from build123d import *

# Parameters (mm, degrees)
SKETCH1_R            = 10.5
BOSS_EXTRUDE1_DEPTH  = 20
SKETCH2_R            = 12
CUT_EXTRUDE1_DEPTH   = 3
SKETCH3_OUTSIDE_W    = 47.968
SKETCH3_OUTSIDE_H    = 58.968
SKETCH3_OUTSIDE_R    = 19
CUT_EXTRUDE2_DEPTH   = 0.25
SKETCH4_OUTSIDE_W    = 47.968
SKETCH4_OUTSIDE_H    = 58.968
SKETCH4_OUTSIDE_R    = 19
CUT_EXTRUDE3_DEPTH   = 0.25
CUT_EXTRUDE4_DEPTH   = 1.5
LPATTERN1_COUNT      = 6
LPATTERN1_PITCH      = 3
MIRROR1_COPY_1_DEPTH = 1.5
MIRROR1_COPY_2_DEPTH = 1.5
MIRROR1_COPY_3_DEPTH = 1.5
MIRROR1_COPY_4_DEPTH = 1.5
MIRROR1_COPY_5_DEPTH = 1.5
CUT_EXTRUDE5_REACH   = 36
SKETCH6_R            = 4
SKETCH7_R            = 1.5
CUT_EXTRUDE6_DEPTH   = 4
SKETCH9_R            = 1.5
CUT_EXTRUDE7_DEPTH   = 6


with BuildPart() as part:
    # Sketch1 → Boss-Extrude1 (new body)
    with BuildSketch(Plane.XY):
        with BuildLine():
            Line((-17, 14.739402973), (-17, -14.739402973))
            ThreePointArc((-17, -14.739402973), (0, -22.5), (17, -14.739402973))
            Line((17, -14.739402973), (17, 14.739402973))
            ThreePointArc((17, 14.739402973), (0, 22.5), (-17, 14.739402973))
        make_face()
        Circle(SKETCH1_R, mode=Mode.SUBTRACT)
    extrude(amount=BOSS_EXTRUDE1_DEPTH)

    # Sketch2 → Cut-Extrude1 (cut)
    with BuildSketch(Plane.XY.offset(20)):
        Circle(SKETCH2_R)
    extrude(amount=-CUT_EXTRUDE1_DEPTH, mode=Mode.SUBTRACT)

    # Sketch3 outside → Cut-Extrude2 (cut)
    with BuildSketch(Plane(origin=(0, 0, 0), x_dir=(-1, 0, 0), z_dir=(0, 0, -1))):
        Rectangle(SKETCH3_OUTSIDE_W, SKETCH3_OUTSIDE_H)
        Circle(SKETCH3_OUTSIDE_R, mode=Mode.SUBTRACT)
    extrude(amount=-CUT_EXTRUDE2_DEPTH, mode=Mode.SUBTRACT)

    # Sketch4 outside → Cut-Extrude3 (cut)
    with BuildSketch(Plane.XY.offset(20)):
        Rectangle(SKETCH4_OUTSIDE_W, SKETCH4_OUTSIDE_H)
        Circle(SKETCH4_OUTSIDE_R, mode=Mode.SUBTRACT)
    extrude(amount=-CUT_EXTRUDE3_DEPTH, mode=Mode.SUBTRACT)

    # Sketch5 → Cut-Extrude4 (cut)
    with BuildSketch(Plane(origin=(0, 0, 1.75), x_dir=(-1, 0, 0), z_dir=(0, 0, -1))):
        with BuildLine():
            Line((17, 8.485281374), (17, 14.739402973))
            ThreePointArc((17, 14.739402973), (0, 22.5), (-17, 14.739402973))
            Line((-17, 14.739402973), (-17, 8.485281374))
            ThreePointArc((-17, 8.485281374), (0, 19), (17, 8.485281374))
        make_face()
    cut_extrude4 = extrude(amount=-CUT_EXTRUDE4_DEPTH, mode=Mode.SUBTRACT)

    # LPattern1: Cut-Extrude4 ×6
    with Locations(*[(0, 0, i * LPATTERN1_PITCH) for i in range(1, LPATTERN1_COUNT)]):
        add(cut_extrude4, mode=Mode.SUBTRACT)

    # Mirror1: Cut-Extrude4 across plane
    add(cut_extrude4.mirror(Plane.ZX), mode=Mode.SUBTRACT)

    # Mirror1 copy 1 sketch → Mirror1 copy 1 (cut)
    with BuildSketch(Plane(origin=(0, 0, 4.75), x_dir=(-1, 0, 0), z_dir=(0, 0, -1))):
        with BuildLine():
            Line((17, -8.485281374), (17, -14.739402973))
            ThreePointArc((17, -14.739402973), (0, -22.5), (-17, -14.739402973))
            Line((-17, -14.739402973), (-17, -8.485281374))
            ThreePointArc((-17, -8.485281374), (0, -19), (17, -8.485281374))
        make_face()
    extrude(amount=-MIRROR1_COPY_1_DEPTH, mode=Mode.SUBTRACT)

    # Mirror1 copy 2 sketch → Mirror1 copy 2 (cut)
    with BuildSketch(Plane(origin=(0, 0, 7.75), x_dir=(-1, 0, 0), z_dir=(0, 0, -1))):
        with BuildLine():
            Line((17, -8.485281374), (17, -14.739402973))
            ThreePointArc((17, -14.739402973), (0, -22.5), (-17, -14.739402973))
            Line((-17, -14.739402973), (-17, -8.485281374))
            ThreePointArc((-17, -8.485281374), (0, -19), (17, -8.485281374))
        make_face()
    extrude(amount=-MIRROR1_COPY_2_DEPTH, mode=Mode.SUBTRACT)

    # Mirror1 copy 3 sketch → Mirror1 copy 3 (cut)
    with BuildSketch(Plane(origin=(0, 0, 10.75), x_dir=(-1, 0, 0), z_dir=(0, 0, -1))):
        with BuildLine():
            Line((17, -8.485281374), (17, -14.739402973))
            ThreePointArc((17, -14.739402973), (0, -22.5), (-17, -14.739402973))
            Line((-17, -14.739402973), (-17, -8.485281374))
            ThreePointArc((-17, -8.485281374), (0, -19), (17, -8.485281374))
        make_face()
    extrude(amount=-MIRROR1_COPY_3_DEPTH, mode=Mode.SUBTRACT)

    # Mirror1 copy 4 sketch → Mirror1 copy 4 (cut)
    with BuildSketch(Plane(origin=(0, 0, 13.75), x_dir=(-1, 0, 0), z_dir=(0, 0, -1))):
        with BuildLine():
            Line((17, -8.485281374), (17, -14.739402973))
            ThreePointArc((17, -14.739402973), (0, -22.5), (-17, -14.739402973))
            Line((-17, -14.739402973), (-17, -8.485281374))
            ThreePointArc((-17, -8.485281374), (0, -19), (17, -8.485281374))
        make_face()
    extrude(amount=-MIRROR1_COPY_4_DEPTH, mode=Mode.SUBTRACT)

    # Mirror1 copy 5 sketch → Mirror1 copy 5 (cut)
    with BuildSketch(Plane(origin=(0, 0, 16.75), x_dir=(-1, 0, 0), z_dir=(0, 0, -1))):
        with BuildLine():
            Line((17, -8.485281374), (17, -14.739402973))
            ThreePointArc((17, -14.739402973), (0, -22.5), (-17, -14.739402973))
            Line((-17, -14.739402973), (-17, -8.485281374))
            ThreePointArc((-17, -8.485281374), (0, -19), (17, -8.485281374))
        make_face()
    extrude(amount=-MIRROR1_COPY_5_DEPTH, mode=Mode.SUBTRACT)

    # Sketch6 → Cut-Extrude5 (cut, up to next)
    with BuildSketch(Plane.ZY.offset(17), mode=Mode.PRIVATE) as cut_extrude5_sk1:
        with Locations((10, 0)):
            Circle(SKETCH6_R)
    cut_extrude5_tool1 = extrude(cut_extrude5_sk1.sketch, amount=-CUT_EXTRUDE5_REACH, mode=Mode.PRIVATE) & part.part
    add(cut_extrude5_tool1.solids().sort_by_distance((-17, 0, 10))[0], mode=Mode.SUBTRACT)

    # Sketch7 → Cut-Extrude6 (cut)
    with BuildSketch(Plane.ZY.offset(17)):
        with Locations((5.050252532, 4.949747468)):
            Circle(SKETCH7_R)
        with Locations((14.949747468, 4.949747468)):
            Circle(SKETCH7_R)
        with Locations((14.949747468, -4.949747468)):
            Circle(SKETCH7_R)
        with Locations((5.050252532, -4.949747468)):
            Circle(SKETCH7_R)
    cut_extrude6 = extrude(amount=-CUT_EXTRUDE6_DEPTH, mode=Mode.SUBTRACT)

    # Sketch8 → Cut-Revolve1 (revolve, cut)
    with BuildSketch(Plane(origin=(0, 0, 10), x_dir=(-1, 0, 0), z_dir=(0, 0, -1))):
        Polygon((-17, 0), (-17, -3), (-14.5, -3), (-11.5, 0), align=None)
    revolve(axis=Axis((11.5, 0, 10), (1, 0, 0)), mode=Mode.SUBTRACT)

    # Mirror2: Cut-Extrude6 across plane
    add(cut_extrude6.mirror(Plane(origin=(0, 0, 0), x_dir=(0, 0, 1), z_dir=(1, 0, 0))), mode=Mode.SUBTRACT)

    # Sketch9 → Cut-Extrude7 (cut)
    with BuildSketch(Plane(origin=(0, 0, 0), x_dir=(-1, 0, 0), z_dir=(0, 0, -1))):
        with Locations((0, 16)):
            Circle(SKETCH9_R)
        with Locations((13.856406461, 8)):
            Circle(SKETCH9_R)
        with Locations((13.856406461, -8)):
            Circle(SKETCH9_R)
        with Locations((0, -16)):
            Circle(SKETCH9_R)
        with Locations((-13.856406461, -8)):
            Circle(SKETCH9_R)
        with Locations((-13.856406461, 8)):
            Circle(SKETCH9_R)
    cut_extrude7 = extrude(amount=-CUT_EXTRUDE7_DEPTH, mode=Mode.SUBTRACT)

    # Mirror3: Cut-Extrude7 across plane
    add(cut_extrude7.mirror(Plane(origin=(0, 0, 10), x_dir=(1, 0, 0), z_dir=(0, 0, -1))), mode=Mode.SUBTRACT)


solid = part.part
Source: CAD feature listing. Evaluate the final solid. Frame: model axes, mm. A direction names the side the tool comes from. Give positions to 0.01 mm unless a question says otherwise; leave off trailing zeros. Write each loop counter-clockwise with the first axis right and the second up, starting at its lowest first coordinate (ties: lowest second). Pieces come first, ordered by that corner, then holes. Notation, with made-up numbers: (52.25, -29.5) -> (65.25, -29.5) arc R26 cw to (65.25, -0.5) -> close; hole circle Ø9 at (1, 73.5). An arc over 180 degrees is marked (long way). Return JSON: item names as keys, results as strings. Group by question number.
1. Pin query (flat end, axial travel): pin 1 Ø2 at (y, z) = (-12.5, 2.5) entering from -X; pin 2 Ø1.5 at (y, z) = (5, 15.5) entering from +X; pin 3 Ø1.8 at (y, z) = (4.95, 14.95) entering from -X; pin 4 Ø1.5 at (x, y) = (0, -15.5) entering from +Z. Return the tip coordinate at first contact, or that it passes through.
2. Section B-B, the plane x = 14. Count the separate pieces of the cut face and the enclosed holes in it, then the cut area to 3 significant figures.
3. Access query for faces 1 (the face through (13, -5, 5)), 2 (the face through (0, 19, 5)), 3 (the face through (0, -20, 19.75)). Directions: +Z, -Z, +X, -X, +Y, -Y. A direction counts if a zero-diameter tool reaches every point of the face in a straight line with its end or side. Return the directions, or none.
4. Section A-A, the plane y = -8. Output: boundary loops of the cut face in (x, z), then the cut area to 3 significant figures.
5. Mould query, pull axis X, two halves, no side actions, for faces 4 (the face through (15.03, 5.4, 16.38)), 5 (the face through (-0.3, -22.5, 16)), 6 (the face through (14, -8, 6)), 7 (the face through (10, 3.2, 8.4)). Classes: +X half, -X half, draft (parallel to the pull), parting line (faces both ways), or undercut.
6. Material intervals for line 1 (X direction, y = -7.5, z = 1.75); line 2 (Y direction, x = 12, z = 2.25); line 3 (Y direction, x = 1, z = 4), sorted ascending. Write a range as from..to.
Determined:
{
 "1": {"pin 1": "stops at x = -17", "pin 2": "stops at x = 13", "pin 3": "stops at x = -13", "pin 4": "stops at z = 14"},
 "2": {"separate pieces": "1", "enclosed holes": "5", "area": "494 mm2"},
 "3": {"face 1": "+X", "face 2": "+Y", "face 3": "+Z, -Y"},
 "4": {"outline": "(-17, 0) -> (-15.36, 0) -> (-15.36, 6) -> (-12.36, 6) -> (-12.36, 0) -> (-6.8, 0) -> (-6.8, 17) -> (-8.94, 17) -> (-8.94, 20) -> (-12.36, 20) -> (-12.36, 14) -> (-15.36, 14) -> (-15.36, 20) -> (-17, 20) -> close; (6.8, 0) -> (12.36, 0) -> (12.36, 6) -> (15.36, 6) -> (15.36, 0) -> (17, 0) -> (17, 20) -> (15.36, 20) -> (15.36, 14) -> (12.36, 14) -> (12.36, 20) -> (8.94, 20) -> (8.94, 17) -> (6.8, 17) -> close", "area": "323 mm2"},
 "5": {"face 4": "draft", "face 5": "parting line", "face 6": "undercut", "face 7": "undercut"},
 "6": {"line 1": "x = -17..-15.27, -12.44..-7.35, 7.35..12.44, 15.27..17", "line 2": "y = -14.73..14.73", "line 3": "y = -22.48..-17.12, -14.88..-10.45, 10.45..14.88, 17.12..22.48"}
}
